Check sheet for the modelled part. Datum: model origin and axes. Units: mm. A direction names the side the tool comes from. Give positions to 0.01 mm unless a question says otherwise; leave off trailing zeros. Write each loop counter-clockwise with the first axis right and the second up, starting at its lowest first coordinate (ties: lowest second). Pieces come first, ordered by that corner, then holes. Notation, with made-up numbers: (43, 45.25) -> (65, 45.25) arc R17 cw to (65, 74.25) -> close; hole circle Ø11 at (-26, 80). An arc over 180 degrees is marked (long way). Use a Markdown table: item, result. Add a question column.
1. Gauge pin test, flat end, axial feed: P1, Ø8, axis at y = 50.5, z = -109, coming from the -X side. Record the tip position at first contact, or that the pin passes through.
2. Cross-section at B-B (x = 37). Enter the section's corners in (y, z), then the cut area to 3 significant figures.
3. Release check for a two-part mould opening along Z. For faces 6 (the flat face through (109, 49, -160)), 7 (the flat face through (69, 1, -56)), 8 (the flat face through (89, 51, -3)) record: released by +Z, released by -Z, zero draft, split by the parting line, or undercut.
4. Cross-section at C-C (y = 22). Enter the section's corners in (x, z), then the cut area to 3 significant figures.
5. Scan lines: probe 1 along Z at (x, y) = (81, 12.5); probe 2 along X at (y, z) = (85, -126.5); probe 3 along X at (y, z) = (47, -51). Record each from-to range of solid material in increasing order. Write a range as [from, to].
6. Cross-section at D-D (y = 76.5). Enter the section's corners in (x, z), then the cut area to 3 significant figures.
7. Set-up check for faces 1 (the flat face through (109, 49, 0)), 2 (the flat face through (3, 83, -79)), 3 (the flat face through (121, 3, -81)), 4 (the flat face through (180, 49, -79)), 5 (the flat face through (177, 51, -79)): record each of +Z, -Z, +X, -X, +Y, -Y from which the full face is reachable in a straight line by a thin tool's end or side.
8. Cross-section at A-A (z = -67). Enter the section's corners in (x, y).
from build123d import *

# Parameters (mm, degrees)
SKETCH1_W               = 180
SKETCH1_H               = 160
BOSS_EXTRUDE1_DEPTH     = 3
SKETCH2_W               = 180
SKETCH2_H               = 160
SKETCH2_W_2             = 174
SKETCH2_H_2             = 154
BOSS_EXTRUDE2_DEPTH     = 100
CUT_EXTRUDE1_DEPTH      = 1
CUT_EXTRUDE1_DEPTH_BACK = 161


with BuildPart() as part:
    # Sketch1 → Boss-Extrude1 (new body)
    with BuildSketch(Plane(origin=(0, 0, 0), x_dir=(1, 0, 0), z_dir=(0, 1, 0))):
        with Locations((90, 80)):
            Rectangle(SKETCH1_W, SKETCH1_H)
    extrude(amount=BOSS_EXTRUDE1_DEPTH)

    # Sketch2 → Boss-Extrude2 (add)
    with BuildSketch(Plane(origin=(0, 0, 0), x_dir=(1, 0, 0), z_dir=(0, 1, 0))):
        with Locations((90, 80)):
            Rectangle(SKETCH2_W, SKETCH2_H)
        with Locations((90, 80)):
            Rectangle(SKETCH2_W_2, SKETCH2_H_2, mode=Mode.SUBTRACT)
    extrude(amount=BOSS_EXTRUDE2_DEPTH)

    # Sketch3 → Cut-Extrude1 (cut, two sides)
    with BuildSketch(Plane.XY) as cut_extrude1_sk:
        Polygon((0, 70), (70, 0), (0, 0), align=None)
    extrude(amount=CUT_EXTRUDE1_DEPTH, mode=Mode.SUBTRACT)
    extrude(cut_extrude1_sk.sketch, amount=-CUT_EXTRUDE1_DEPTH_BACK, mode=Mode.SUBTRACT)


solid = part.part
Worked answers:
| question | item | result |
|---|---|---|
| 1 | P1 | stops at x = 177 |
| 2 | outline | (33, -160) -> (100, -160) -> (100, -157) -> (33, -157) -> close; (33, -3) -> (100, -3) -> (100, 0) -> (33, 0) -> close |
| 2 | area | 402 mm² |
| 3 | face 6 | released by -Z |
| 3 | face 7 | zero draft |
| 3 | face 8 | undercut |
| 4 | outline | (48, -160) -> (180, -160) -> (180, 0) -> (48, 0) -> (48, -3) -> (177, -3) -> (177, -157) -> (48, -157) -> close |
| 4 | area | 1,250 mm² |
| 5 | probe 1 | z = [-160, -157], [-3, 0] |
| 5 | probe 2 | x = [0, 3], [177, 180] |
| 5 | probe 3 | x = [177, 180] |
| 6 | outline | (0, -160) -> (180, -160) -> (180, 0) -> (0, 0) -> close; hole (3, -157) -> (177, -157) -> (177, -3) -> (3, -3) -> close |
| 6 | area | 2,000 mm² |
| 7 | face 1 | +Z, +X, -X, +Y, -Y |
| 7 | face 2 | +Y, -Y |
| 7 | face 3 | -X, +Y |
| 7 | face 4 | +Z, -Z, +X, +Y, -Y |
| 7 | face 5 | +Y |
| 8 | outline | (0, 70) -> (3, 67) -> (3, 100) -> (0, 100) -> close; (67, 3) -> (70, 0) -> (180, 0) -> (180, 100) -> (177, 100) -> (177, 3) -> close |
